Geometry check sheet. Reference: the model listing, model coordinates, mm. A direction names the side the tool comes from. Coordinates: 2 decimals unless noted, no trailing zeros. Order: outer loops, then holes, each group sorted by start corner. A loop starts at its lowest first (then second) coordinate and runs counter-clockwise, first axis right, second up. Notation, with made-up numbers: (14.5, 10.5) - (34.5, 10.5) arc R14 cw to (34.5, 19.5) - close; hole circle Ø2 at (88.25, 29.5). An arc over 180 degrees is marked (long way). Put each result on its own line as item: value.
from build123d import *

# Parameters (mm, degrees)
SKETCH1_W           = 100
SKETCH1_H           = 50
BOSS_EXTRUDE1_DEPTH = 30
SKETCH3_R           = 23.162771803
BOSS_EXTRUDE2_DEPTH = 70
SKETCH4_R           = 23.656320331
BOSS_EXTRUDE3_DEPTH = 200
SKETCH5_R           = 8.525466093
BOSS_EXTRUDE4_DEPTH = 400


with BuildPart() as part:
    # Sketch1 → Boss-Extrude1 (new body)
    with BuildSketch(Plane(origin=(0, 0, 0), x_dir=(1, 0, 0), z_dir=(0, 1, 0))):
        Rectangle(SKETCH1_W, SKETCH1_H)
    extrude(amount=BOSS_EXTRUDE1_DEPTH)

    # Sketch3 → Boss-Extrude2 (add)
    with BuildSketch(Plane(origin=(0, 30, 0), x_dir=(1, 0, 0), z_dir=(0, 1, 0))):
        with Locations(Location((-24.62884077, 0, 0), (0, 0, 270))):
            Circle(SKETCH3_R)
    extrude(amount=BOSS_EXTRUDE2_DEPTH)

    # Sketch4 → Boss-Extrude3 (add)
    with BuildSketch(Plane(origin=(0, 30, 0), x_dir=(1, 0, 0), z_dir=(0, 1, 0))):
        with Locations(Location((24.089523089, 0, 0), (0, 0, 270))):
            Circle(SKETCH4_R)
    extrude(amount=BOSS_EXTRUDE3_DEPTH)

    # Sketch5 → Boss-Extrude4 (add)
    with BuildSketch(Plane(origin=(0, 230, 0), x_dir=(1, 0, 0), z_dir=(0, 1, 0))):
        with Locations(Location((24.089523089, 0, 0), (0, 0, 270))):
            Circle(SKETCH5_R)
    extrude(amount=BOSS_EXTRUDE4_DEPTH)


solid = part.part
Q1. Section check A-A on z = 0. Record the boundary of the cut face in (x, y), then the cut area to 3 significant figures.
Answer block:
outline: (-50, 0) - (50, 0) - (50, 30) - (47.75, 30) - (47.75, 230) - (32.61, 230) - (32.61, 630) - (15.56, 630) - (15.56, 230) - (0.43, 230) - (0.43, 30) - (-1.47, 30) - (-1.47, 100) - (-47.79, 100) - (-47.79, 30) - (-50, 30) - close
area: 22,500 mm^2
Q2. Section check C-C on y = 528. Record the boundary of the cut face in (x, z).
Answer block:
outline: circle Ø17.05 at (24.09, 0)
Q3. Thickness scan on L1, parallel to Y at x = 9, z = -8; L2, parallel to X at y = 52, z = -8; L3, parallel to Y at x = -19.5, z = 0. Record the ranges inside material, lowest first. Write a range as [from, to].
Answer block:
L1: y = [0, 230]
L2: x = [-46.37, -2.89], [1.83, 46.35]
L3: y = [0, 100]
Q4. Depth check by flat-ended pin: pin 1 Ø1.5 at (x, z) = (25.5, 17) entering from -Y; pin 2 Ø1 at (x, z) = (21, -18.5) entering from +Y; pin 3 Ø12 at (x, z) = (-33.5, -1) entering from +Y; pin 4 Ø8 at (x, y) = (-34, 102) entering from +Z. Enter the tip coordinate at first touch or a pass-through.
Answer block:
pin 1: stops at y = 0
pin 2: stops at y = 230
pin 3: stops at y = 100
pin 4: stops at z = 22.4
Q5. Access from +Z, -Z, +X, -X, +Y, -Y to the whole of each face (thin tool, end or side, straight path). Record for faces 1 (the cylindrical face through (0.996, 128.6, -5.128)), 2 (the flat face through (-24, 100, 0)), 3 (the flat face through (-1, 15, -25)).
Answer block:
face 1: +Y
face 2: +Z, -Z, -X, +Y
face 3: -Z, +X, -X, +Y, -Y
Q6. Section check B-B on x = -17. Record the boundary of the cut face in (y, z), then the cut area to 3 significant figures.
Answer block:
outline: (0, -25) - (30, -25) - (30, -21.87) - (100, -21.87) - (100, 21.87) - (30, 21.87) - (30, 25) - (0, 25) - close
area: 4,560 mm^2
